Here's how the part is built. I have some questions about the finished solid (model axes, mm). A direction names the side the tool comes from. Coordinates: 2 decimals unless noted, no trailing zeros. Order: outer loops, then holes, each group sorted by start corner. A loop starts at its lowest first (then second) coordinate and runs counter-clockwise, first axis right, second up. Notation, with made-up numbers: (85, 13) - (109, 13) arc R27 cw to (109, 35) - close; hole circle Ø5 at (52.5, 30.5). An arc over 180 degrees is marked (long way). Answer in a Markdown table with one row per item. Add a question column.
Item 1: If I drill on line 1 along Y through (x, z) = (0, 24); line 2 along Y through (x, z) = (0, 13.5); line 3 along X through (y, z) = (3, 19.5), over which ranges is the centre line in solid material (lowest first)? Write a range as from..to.
Item 2: On a 3-axis mill with a long thin cutter (end or side, diameter ignored), from which of +Z, -Z, +X, -X, +Y, -Y can I reach the whole of each face in a straight line? I mean faces 4 (the cylindrical face through (-3.78, -2.9, 23.55)), 5 (the flat face through (0, 0, 17.78)), 6 (the flat face through (0, 2, 0)). Say none if no direction works.
Item 3: Thinking about a two-plate mould opening in Y: for faces 1 (the flat face through (0, 0, 18.725)), 2 (the flat face through (0, 5, 28.25)), 3 (the conical face through (-17.243, 13.222, 18.422)), which applies, +Y half, -Y half, draft (parallel to the pull), parting line (faces both ways), or undercut?
Item 4: I want a section at C-C (z = 24.5). Please give me the cut outline in (x, y) (1 decimal).
Item 5: I want a section at D-D (z = 10.75). Please give me the cut outline in (x, y) (1 decimal).
Item 6: Will these pins go through, and if not, where does the flat tip stop? pin 1 Ø12 at (x, y) = (11, -15) entering from +Z; pin 2 Ø1 at (x, z) = (-6.5, 18.5) entering from -Y; pin 3 Ø2 at (x, z) = (-11, 24) entering from +Y; pin 4 Ø3 at (x, y) = (-2, 1.5) entering from +Z.
```python
from build123d import *

# Parameters (mm, degrees)
F2_R     = 4.7625
F3_DEPTH = 9.525
F4_R     = 1.5875
F5_DEPTH = 17.78


with BuildPart() as f1:
    # F0 (on Front) → F1 (revolve)
    with BuildSketch(Plane.XZ):
        with BuildLine():
            Line((12.743474, 20.729434), (5.371063, 22.575061))
            Line((5.371063, 22.575061), (5.371063, 28.250467))
            Line((5.371063, 28.250467), (0, 28.250467))
            Line((0, 28.250467), (0, 0))
            Line((0, 0), (2.540102, 0))
            Line((2.540102, 0), (4.674008, 2.74161))
            Line((4.674008, 2.74161), (12.14571, 2.74161))
            ThreePointArc((12.14571, 2.74161), (13.167332, 2.824331), (14.162337, 3.070338))
            Line((14.162337, 3.070338), (27.477805, 7.529916))
            ThreePointArc((27.477805, 7.529916), (28.234492, 8.290196), (28.078277, 9.351419))
            Line((28.078277, 9.351419), (21.404842, 18.884539))
            ThreePointArc((21.404842, 18.884539), (20.61201, 19.617126), (19.586547, 19.954304))
            Line((19.586547, 19.954304), (13.62924, 20.573351))
            ThreePointArc((13.62924, 20.573351), (13.18359, 20.63569), (12.743474, 20.729434))
        make_face()
    revolve(axis=Axis((0, 0, 14.125234), (0, 0, -1)))

    # F2 (on face) → F3 (cut)
    with BuildSketch(Plane.XY.offset(28.250467)):
        Circle(F2_R)
    extrude(amount=-F3_DEPTH, mode=Mode.SUBTRACT)

    # F4 (on face) → F5 (cut)
    with BuildSketch(Plane(origin=(0, 0, 0), x_dir=(1, 0, 0), z_dir=(0, 0, -1))):
        Circle(F4_R)
    extrude(amount=-F5_DEPTH, mode=Mode.SUBTRACT)


solid = f1.part
```
Values follow:
| question | item | result |
|---|---|---|
| 1 | line 1 | y = -5.37..-4.76, 4.76..5.37 |
| 1 | line 2 | y = -25.17..-1.59, 1.59..25.17 |
| 1 | line 3 | x = -20.58..-3.7, 3.7..20.58 |
| 2 | face 4 | +Z |
| 2 | face 5 | -Z |
| 2 | face 6 | -Z, +X, -X, +Y, -Y |
| 3 | face 1 | undercut |
| 3 | face 2 | draft |
| 3 | face 3 | parting line |
| 4 | outline | circle Ø10.7 at (0, 0); hole circle Ø9.5 at (0, 0) |
| 5 | outline | circle Ø54.2 at (0, 0); hole circle Ø3.2 at (0, 0) |
| 6 | pin 1 | stops at z = 20.77 |
| 6 | pin 2 | stops at y = -21.07 |
| 6 | pin 3 | passes through |
| 6 | pin 4 | stops at z = 18.73 |
